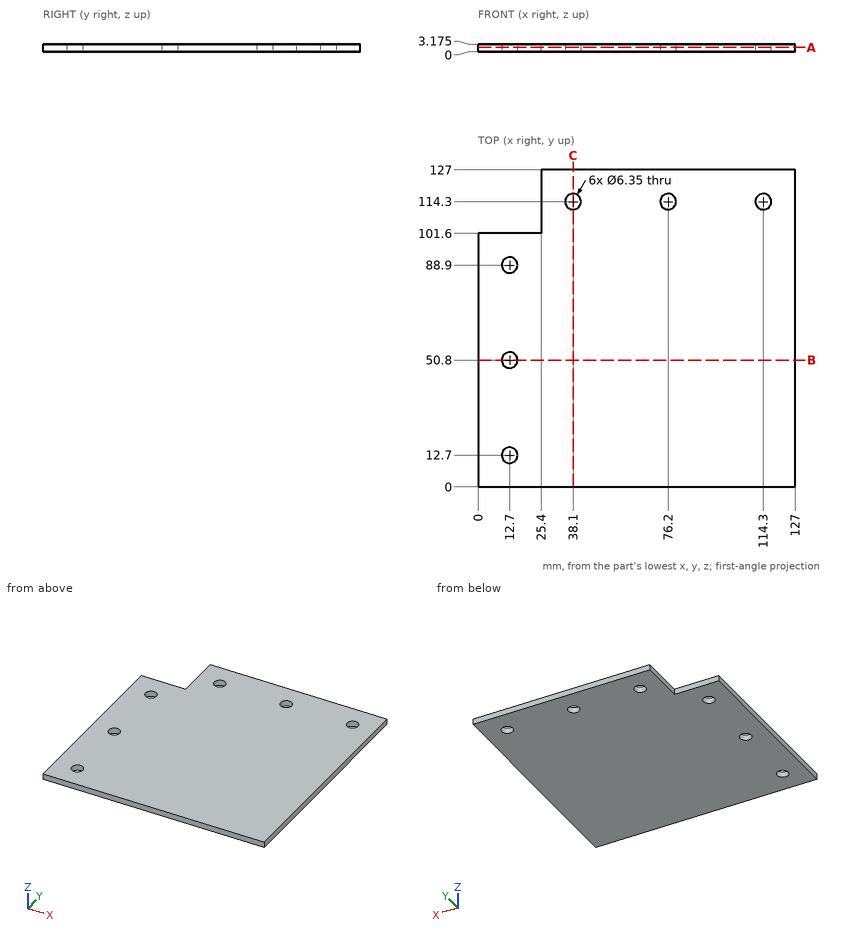
Geometry check sheet. Reference: drawing and pictorial views, mm from the part's lowest x, y, z. Give positions to 0.01 mm unless a question says otherwise; leave off trailing zeros. Order: outer loops, then holes, each group sorted by start corner. A loop starts at its lowest first (then second) coordinate and runs counter-clockwise, first axis right, second up. Notation, with made-up numbers: M 62.25,-23 L 102.25,-23 A25 cw 102.25,-11 Z; hole C -2,33.25 d6. An arc over 180 degrees is marked long. Answer in a Markdown table with one row per item.
1) Cross-section at B-B, the plane y = 50.8. Enter the section's corners in (x, z) (3 decimals), plus the area to 3 significant figures.
Filled sheet:
| item | result |
|---|---|
| outline | M 0,0 L 9.525,0 L 9.525,3.175 L 0,3.175 Z; M 15.875,0 L 127,0 L 127,3.175 L 15.875,3.175 Z |
| area | 383 mm2 |
2) Gauge pin test, flat ends, axial feed: P1, Ø1.5, axis at y = 92.5, z = 1.5, coming from the -X side; P2, Ø1, axis at x = 16.5, z = 1, coming from the +Y side. Record the tip position at first contact, or that the pin passes through.
Filled sheet:
| item | result |
|---|---|
| P1 | stops at x = 0 |
| P2 | stops at y = 101.6 |
3) Cross-section at C-C, the plane x = 38.1. Enter the section's corners in (y, z) (3 decimals), plus the area to 3 significant figures.
Filled sheet:
| item | result |
|---|---|
| outline | M 0,0 L 111.125,0 L 111.125,3.175 L 0,3.175 Z; M 117.475,0 L 127,0 L 127,3.175 L 117.475,3.175 Z |
| area | 383 mm2 |
4) Cross-section at A-A, the plane z = 1.8. Enter the section's corners in (x, y) (3 decimals), plus the area to 3 significant figures.
Filled sheet:
| item | result |
|---|---|
| outline | M 0,0 L 127,0 L 127,127 L 25.4,127 L 25.4,101.6 L 0,101.6 Z; hole C 12.7,12.7 d6.35; hole C 12.7,50.8 d6.35; hole C 12.7,88.9 d6.35; hole C 38.1,114.3 d6.35; hole C 76.2,114.3 d6.35; hole C 114.3,114.3 d6.35 |
| area | 15,300 mm2 |
5) Thickness scan on L1, parallel to Y at x = 12.7, z = 2 (3 decimals); L2, parallel to Y at x = 114, z = 0.9; L3, parallel to Y at x = 117, z = 1.7. Record the ranges inside material, lowest first. Write a range as [from, to].
Filled sheet:
| item | result |
|---|---|
| L1 | y = [0, 9.525], [15.875, 47.625], [53.975, 85.725], [92.075, 101.6] |
| L2 | y = [0, 111.14], [117.46, 127] |
| L3 | y = [0, 112.63], [115.97, 127] |
